Answer from the drawing. Dimensions are ordinates in mm from the lowest x, y and z of the part. Coordinates: 2 decimals unless noted, no trailing zeros. Write each loop counter-clockwise with the first axis right and the second up, starting at its lowest first coordinate (ties: lowest second). Pieces come first, ordered by that corner, then holes.
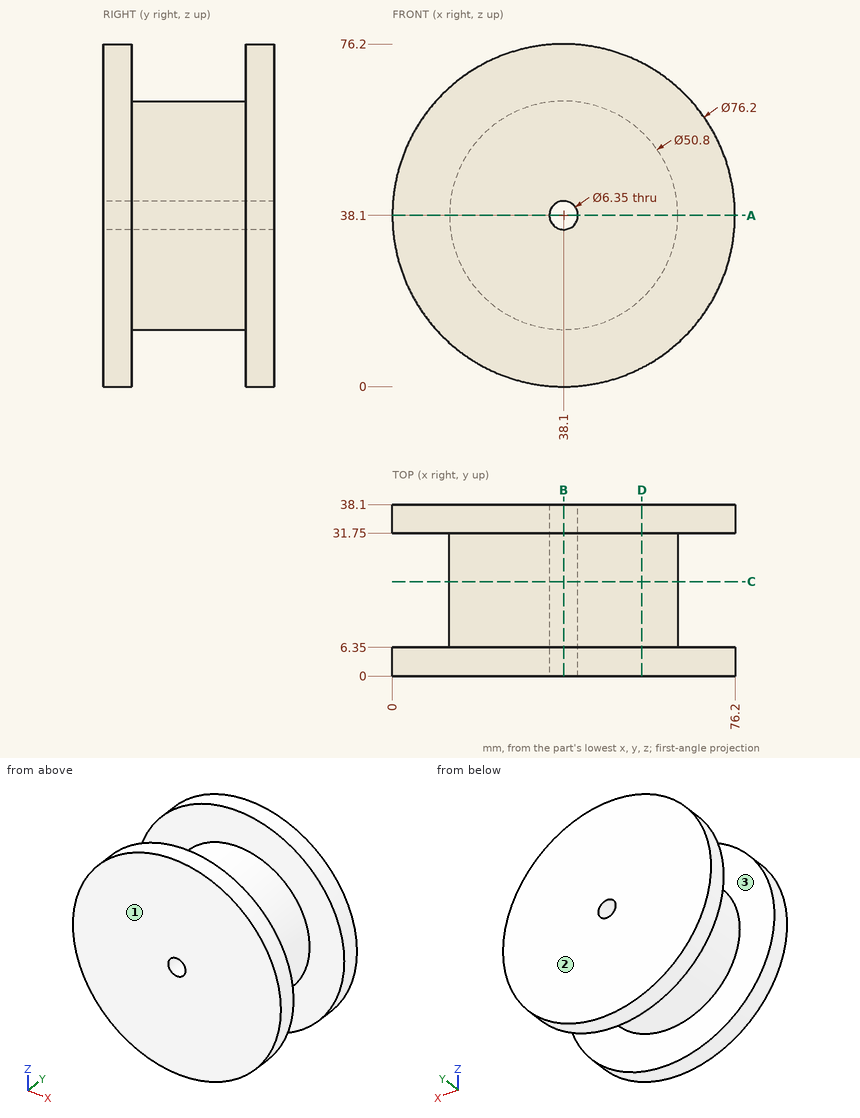
(1) Section B-B, the plane x = 38.1 is taken. Write down the section's boundary in (y, z) (3 decimals), plus the area to 3 significant figures.
(2) For a pull along Y with two mould halves and no side action, classify the marked faces 1, 2 and 3 as pulls with the +Y half, pulls with the -Y half, needs draft (parallel to the pull), parting line crosses it, or undercut.
(3) Section C-C, the plane y = 21 is taken. Write down the section's boundary in (x, z) (3 decimals), plus the area to 3 significant figures.
(4) Section D-D, the plane x = 55.5 is taken. Write down the section's boundary in (y, z).
(5) Each of these flat-tipped pins is pushed along its axis until it touches: pin 1 (6 mm diameter, centred on y = 10, z = 38.5, fed in from -X); pin 2 (3 mm diameter, centred on x = 31.5, y = 22.5, fed in from -Z); pin 3 (1 mm diameter, centred on x = 49.5, y = 34, fed in from -Z). Where does it stop, or does it pass through?
(6) Section A-A, the plane z = 38.1 is taken. Write down the section's boundary in (x, y) (3 decimals), plus the area to 3 significant figures.
(7) Find the intervals of material crossed by probe 1 along Z at (x, y) = (38.1, 23) (3 decimals); probe 2 along Y at (x, z) = (48, 68); probe 3 along X at (y, z) = (3, 35.5), in increasing order.
Solution:
1. outline: (0, 0) - (6.35, 0) - (6.35, 12.7) - (31.75, 12.7) - (31.75, 0) - (38.1, 0) - (38.1, 34.925) - (0, 34.925) - close; (0, 41.275) - (38.1, 41.275) - (38.1, 76.2) - (31.75, 76.2) - (31.75, 63.5) - (6.35, 63.5) - (6.35, 76.2) - (0, 76.2) - close
1. area: 2,020 mm2
2. face 1: pulls with the -Y half
2. face 2: pulls with the +Y half
2. face 3: undercut
3. outline: circle Ø50.8 at (38.1, 38.1); hole circle Ø6.35 at (38.1, 38.1)
3. area: 2,000 mm2
4. outline: (0, 4.21) - (6.35, 4.21) - (6.35, 19.6) - (31.75, 19.6) - (31.75, 4.21) - (38.1, 4.21) - (38.1, 71.99) - (31.75, 71.99) - (31.75, 56.6) - (6.35, 56.6) - (6.35, 71.99) - (0, 71.99) - close
5. pin 1: stops at x = 12.7
5. pin 2: stops at z = 13.22
5. pin 3: stops at z = 1.59
6. outline: (0, 0) - (34.925, 0) - (34.925, 38.1) - (0, 38.1) - (0, 31.75) - (12.7, 31.75) - (12.7, 6.35) - (0, 6.35) - close; (41.275, 0) - (76.2, 0) - (76.2, 6.35) - (63.5, 6.35) - (63.5, 31.75) - (76.2, 31.75) - (76.2, 38.1) - (41.275, 38.1) - close
6. area: 2,020 mm2
7. probe 1: z = 12.7 to 34.925, 41.275 to 63.5
7. probe 2: y = 0 to 6.35, 31.75 to 38.1
7. probe 3: x = 0.09 to 36.28, 39.92 to 76.11
